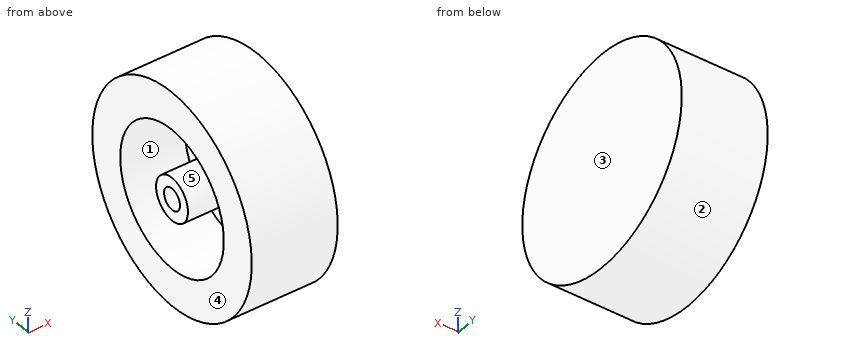
```python
from build123d import *

# Parameters (mm, degrees)
SKETCH_1_R          = 10
EXTRUDE_1_DEPTH     = 4
SKETCH_2_R          = 6.5
SKETCH_2_R_2        = 2
SKETCH_2_R_3        = 1
CUT_EXTRUDE_1_DEPTH = 6


with BuildPart() as part:
    # 草图1 → 凸台-拉伸1 (new, symmetric)
    with BuildSketch(Plane(origin=(0, 0, 0), x_dir=(0, 0, -1), z_dir=(1, 0, 0))):
        Circle(SKETCH_1_R)
    extrude(amount=EXTRUDE_1_DEPTH, both=True)

    # 草图2 → 切除-拉伸1 (cut)
    # profile 1 of 2: a face of its own
    with BuildSketch(Plane.ZY.offset(4)):
        Circle(SKETCH_2_R)
        Circle(SKETCH_2_R_2, mode=Mode.SUBTRACT)
    # profile 2 of 2: a face of its own
    with BuildSketch(Plane.ZY.offset(4)):
        Circle(SKETCH_2_R_3)
    extrude(amount=-CUT_EXTRUDE_1_DEPTH, mode=Mode.SUBTRACT)


solid = part.part
```
Build history of the part. All positions in model axes, mm. Face numbers are marked on the shaded views. A direction names the side the tool comes from. Coordinates: 2 decimals unless noted, no trailing zeros. Order: outer loops, then holes, each group sorted by start corner. A loop starts at its lowest first (then second) coordinate and runs counter-clockwise, first axis right, second up.
Item 1: Mould opens along Y. For the marked faces 1, 2 and 3 say: released by +Y, released by -Y, zero draft, split by the parting line, or undercut.
Filled in:
face 1: undercut
face 2: split by the parting line
face 3: zero draft
Item 2: Saw through at C-C on x = 0.25. List the corners of the cut face in (y, z), then the cut area to 3 significant figures.
Filled in:
outline: circle Ø20 at (0, 0); circle Ø4 at (0, 0); hole circle Ø13 at (0, 0); hole circle Ø2 at (0, 0)
area: 191 mm2
Item 3: Saw through at D-D on y = 6.25. List the corners of the cut face in (x, z), then the cut area to 3 significant figures.
Filled in:
outline: (-4, -7.81) - (4, -7.81) - (4, 7.81) - (-4, 7.81) - (-4, 1.79) - (2, 1.79) - (2, -1.79) - (-4, -1.79) - close
area: 103 mm2
Item 4: Tool access for the marked faces 4 and 5: list every direction of +Z, -Z, +X, -X, +Y, -Y with a clear straight run to the whole face (end or side of a thin tool).
Filled in:
face 4: +Z, -Z, -X, +Y, -Y
face 5: -X
Item 5: Drill centre lines: L1, parallel to Y at x = -2.3, z = 0; L2, parallel to X at y = -1.25, z = 1.75; L3, parallel to Z at x = -1.5, y = 3.25. Where is each one in solid material? Low to high.
Filled in:
L1: y = -10 to -6.5, -2 to -1, 1 to 2, 6.5 to 10
L2: x = 2 to 4
L3: z = -9.46 to -5.63, 5.63 to 9.46
Item 6: Saw through at A-A on z = 0. List the corners of the cut face in (x, y).
Filled in:
outline: (-4, -10) - (4, -10) - (4, 10) - (-4, 10) - (-4, 6.5) - (2, 6.5) - (2, 2) - (-4, 2) - (-4, 1) - (2, 1) - (2, -1) - (-4, -1) - (-4, -2) - (2, -2) - (2, -6.5) - (-4, -6.5) - close
Item 7: Drop flat-ended pins along their axis: pin 1 Ø1.5 at (x, y) = (-0.5, -7) entering from +Z; pin 2 Ø2 at (x, z) = (1, -2) entering from +Y; pin 3 Ø4 at (x, y) = (1.5, -5.5) entering from -Z. Give the stop position or say it passes through.
Filled in:
pin 1: stops at z = 7.81
pin 2: stops at y = 9.95
pin 3: stops at z = -9.37
